The listing builds one solid part. Answer for the finished solid, in the listing's coordinates (mm). Face numbers are marked on the shaded views. A direction names the side the tool comes from. Round coordinates to 2 decimals unless told otherwise and drop trailing zeros. Loops run counter-clockwise (first coordinate to the right, second up) from the corner with the lowest first, then second, coordinate; pieces in that order, holes last. Notation, with made-up numbers: (89, 67) -> (128, 67) arc R31 ccw to (128, 105) -> close; hole circle Ø5 at (34.25, 80.5). An arc over 180 degrees is marked (long way). Answer in a Markdown table with one row per item. Add a question column.
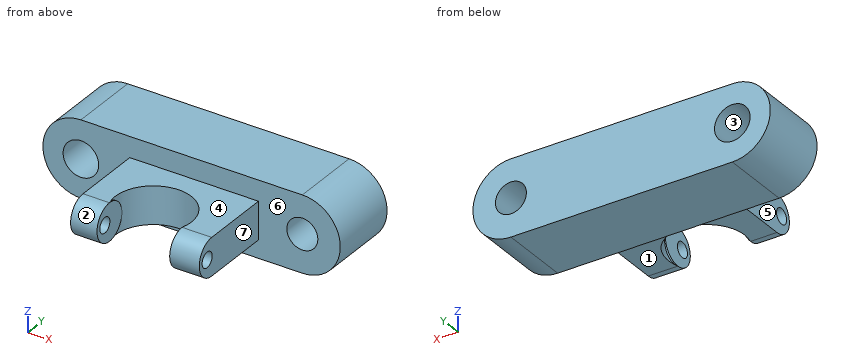
```python
from build123d import *

# Parameters (mm, degrees)
F0_R      = 6.3984297888
F0_R_2    = 5.5753
F1_DEPTH  = 25.4
F2_W      = 46.2799873203
F2_H      = 13.5046518408
F3_DEPTH  = 25.4
F5_DEPTH  = 69.342
F6_W      = 9.5002483577
F6_H      = 6.7523259204
F7_W      = 10.6321182102
F7_H      = 6.7523259204
F10_R     = 2.7327204499
F11_DEPTH = 182.626


with BuildPart() as f1:
    # F0 (on Front) → F1 (new body)
    with BuildSketch(Plane.XZ):
        with BuildLine():
            Line((43.7605383081, 27.3248670252), (-35.8691346556, 27.3248670252))
            ThreePointArc((-35.8691346556, 27.3248670252), (-49.5315681682, 13.6624335126), (-35.8691346556, 0))
            Line((-35.8691346556, 0), (43.7605383081, 0))
            ThreePointArc((43.7605383081, 0), (57.4229718207, 13.6624335126), (43.7605383081, 27.3248670252))
        make_face()
        with Locations((-35.8691346556, 13.6624335126)):
            Circle(F0_R, mode=Mode.SUBTRACT)
        with Locations((43.7605383081, 13.6624335126)):
            Circle(F0_R_2, mode=Mode.SUBTRACT)
    extrude(amount=F1_DEPTH)

    # F2 (on face) → F3 (join)
    with BuildSketch(Plane.XZ.offset(25.4)):
        with Locations((4.8549743369, 13.1856810767)):
            Rectangle(F2_W, F2_H)
    extrude(amount=F3_DEPTH)

    # F4 (on face) → F5 (cut)
    with BuildSketch(Plane(origin=(0, 0, 6.4333551563), x_dir=(1, 0, 0), z_dir=(0, 0, -1))):
        with BuildLine():
            Line((17.3628497869, 50.8), (-8.7847709656, 50.8))
            ThreePointArc((-8.7847709656, 50.8), (4.2890394107, 33.0230943258), (17.3628497869, 50.8))
        make_face()
    extrude(amount=-F5_DEPTH, mode=Mode.SUBTRACT)

    # F6 (on face) → F8 (revolve)
    with BuildSketch(Plane.XZ.offset(50.8)):
        with Locations((-13.5348951444, 9.8095181165)):
            Rectangle(F6_W, F6_H)
    revolve(axis=Axis((-13.5348951444, -50.8, 13.1856810767), (1, 0, 0)))

    # F7 (on face) → F9 (revolve)
    with BuildSketch(Plane.XZ.offset(50.8)):
        with Locations((22.678908892, 9.8095181165)):
            Rectangle(F7_W, F7_H)
    revolve(axis=Axis((22.678908892, -50.8, 13.1856810767), (1, 0, 0)))

    # F10 (on face) → F11 (cut)
    with BuildSketch(Plane.YZ.offset(27.9949679971)):
        with Locations((-53.2889179885, 13.3134396747)):
            Circle(F10_R)
    extrude(amount=-F11_DEPTH, mode=Mode.SUBTRACT)


solid = f1.part
```
Item 1: For the marked faces 4, 5, 6 and 7, determine the directions among +Z, -Z, +X, -X, +Y, -Y from which every point of the face is accessible in a straight line to the end or side of a thin tool.
Item 2: Section C-C, the plane x = 32 is taken. Write down the section's boundary in (y, z).
Item 3: Section A-A, the plane y = -19 is taken. Write down the section's boundary in (x, z).
Item 4: Section B-B, the plane y = -54 is taken. Write down the section's boundary in (x, z).
Item 5: The mould has two halves that part along Z. Classify the marked faces 1, 2 and 3: +Z half, -Z half, draft (parallel to the pull), parting line (faces both ways), or undercut.
Item 6: Flat-ended cylindrical pins translate along their axes: P1, Ø3.5, axis at y = -53.29, z = 13.31, coming from the -X side; P2, Ø6, axis at y = -23.5, z = 18, coming from the +X side; P3, Ø20.5, axis at x = -6.5, y = -37, coming from the +Z side; P4, Ø3, axis at y = -22.5, z = 20, coming from the +X side. Find the tip coordinate at first contact, or state that the pin passes through.
Item 7: Section D-D, the plane z = 5.25 is taken. Write down the section's boundary in (x, y), and give its area (3 significant figures).
Item 8: Consider L1, parallel to X at y = -15.5, z = 12.75; L2, parallel to Z at x = 43.5, y = -15.5; L3, parallel to X at y = -16.5, z = 10.75. Determine where each line is inside the solid, lowest interval first. Write a range as from..to.
Here are the results:
| question | item | result |
|---|---|---|
| 1 | face 4 | +Z, +X, -X, -Y |
| 1 | face 5 | +Z, -Z, -X, -Y |
| 1 | face 6 | -Y |
| 1 | face 7 | +Z, -Z, +X, -Y |
| 2 | outline | (-25.4, 0) -> (0, 0) -> (0, 27.32) -> (-25.4, 27.32) -> close |
| 3 | outline | (-35.87, 0) -> (43.76, 0) arc R13.66 ccw to (43.76, 27.32) -> (-35.87, 27.32) arc R13.66 ccw to start; hole circle Ø12.8 at (-35.87, 13.66); hole circle Ø11.15 at (43.76, 13.66) |
| 4 | outline | (-18.29, 7.24) -> (-8.78, 7.24) -> (-8.78, 10.67) -> (-18.29, 10.67) -> close; (-18.29, 15.95) -> (-8.78, 15.95) -> (-8.78, 19.13) -> (-18.29, 19.13) -> close; (17.36, 7.24) -> (27.99, 7.24) -> (27.99, 10.67) -> (17.36, 10.67) -> close; (17.36, 15.95) -> (27.99, 15.95) -> (27.99, 19.13) -> (17.36, 19.13) -> close |
| 5 | face 1 | -Z half |
| 5 | face 2 | parting line |
| 5 | face 3 | undercut |
| 6 | P1 | passes through |
| 6 | P2 | stops at x = 57.36 |
| 6 | P3 | stops at z = 19.94 |
| 6 | P4 | stops at x = 56.54 |
| 7 | outline | (-46.63, -25.4) -> (54.53, -25.4) -> (54.53, 0) -> (-46.63, 0) -> close |
| 7 | area | 2,570 mm² |
| 8 | L1 | x = -49.5..-42.2, -29.54..38.26, 49.26..57.39 |
| 8 | L2 | z = 0..8.09, 19.23..27.32 |
| 8 | L3 | x = -49.22..-41.57, -30.17..39.01, 48.51..57.11 |
